```python
from build123d import *

# Parameters (mm, degrees)
F1_DEPTH = 6.858


with BuildPart() as f1:
    # F0 (on Front) → F1 (new body)
    with BuildSketch(Plane.XZ):
        with BuildLine():
            Line((28.575, 3.175), (0, 3.175))
            Line((0, 3.175), (-28.575, 3.175))
            ThreePointArc((-28.575, 3.175), (-48.6519, 5.867462), (-67.31, 13.754578))
            Line((-67.31, 13.754578), (-91.44, 13.754578))
            Line((-91.44, 13.754578), (-91.44, -13.754578))
            Line((-91.44, -13.754578), (-67.31, -13.754578))
            ThreePointArc((-67.31, -13.754578), (-48.6519, -5.867462), (-28.575, -3.175))
            Line((-28.575, -3.175), (0, -3.175))
            Line((0, -3.175), (28.575, -3.175))
            ThreePointArc((28.575, -3.175), (48.6519, -5.867462), (67.31, -13.754578))
            Line((67.31, -13.754578), (91.44, -13.754578))
            Line((91.44, -13.754578), (91.44, 13.754578))
            Line((91.44, 13.754578), (67.31, 13.754578))
            ThreePointArc((67.31, 13.754578), (48.6519, 5.867462), (28.575, 3.175))
        make_face()
    extrude(amount=F1_DEPTH)


solid = f1.part
```
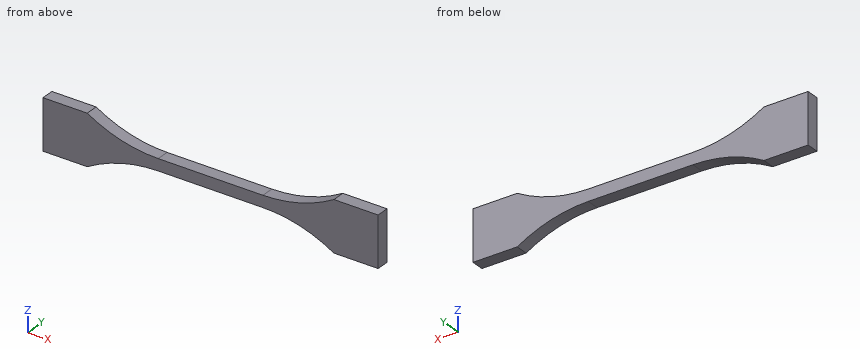
CAD build for the part. Positions are in the model's coordinates, mm. Round coordinates to 2 decimals unless told otherwise and drop trailing zeros. Loops run counter-clockwise (first coordinate to the right, second up) from the corner with the lowest first, then second, coordinate; pieces in that order, holes last. Notation, with made-up numbers: M 40,-32.5 L 88,-32.5 A23 ccw 88,-5.5 Z; hole C 10.25,-23 d8. An arc over 180 degrees is marked long. Return JSON: item names as keys, results as strings. Group by question number.
(1) Saw through at C-C, the plane x = -18. List the corners of the cut face in (y, z) (3 decimals).
(2) Drop flat-ended pins along their axis: P1, Ø1, axis at x = -2, z = 3.5, coming from the +Y side; P2, Ø10, axis at x = 37, z = -10, coming from the -Y side; P3, Ø4, axis at x = 11.5, y = -2.5, coming from the -Z side (3 decimals). Give the stop position or say it passes through.
(3) Saw through at D-D, the plane z = -10.5. List the corners of the cut face in (x, y), and give its area (3 significant figures).
(4) Saw through at A-A, the plane z = 8.5. List the corners of the cut face in (x, y), and give its area (3 significant figures).
(5) Wall check: probe 1 along X at (y, z) = (-1.5, -9.5); probe 2 along X at (y, z) = (-1.5, 10.75); probe 3 along Z at (x, y) = (15, -0.75) (3 decimals). Give the ranges that are in metal, low to high. Write a range as [from, to].
(6) Saw through at B-B, the plane y = -1.25. List the corners of the cut face in (x, z) (3 decimals), and give its area (3 significant figures).
Answer list:
{
 "1": {"outline": "M -6.858,-3.175 L 0,-3.175 L 0,3.175 L -6.858,3.175 Z"},
 "2": {"P1": "y = 0", "P2": "through", "P3": "z = -3.175"},
 "3": {"outline": "M -91.44,-6.86 L -61.17,-6.86 L -61.17,0 L -91.44,0 Z; M 61.17,-6.86 L 91.44,-6.86 L 91.44,0 L 61.17,0 Z", "area": "415 mm2"},
 "4": {"outline": "M -91.44,-6.86 L -56.56,-6.86 L -56.56,0 L -91.44,0 Z; M 56.56,-6.86 L 91.44,-6.86 L 91.44,0 L 56.56,0 Z", "area": "478 mm2"},
 "5": {"probe 1": "[-91.44, -58.97], [58.97, 91.44]", "probe 2": "[-91.44, -61.7], [61.7, 91.44]", "probe 3": "[-3.175, 3.175]"},
 "6": {"outline": "M -91.44,-13.755 L -67.31,-13.755 A76.2 cw -28.575,-3.175 L 28.575,-3.175 A76.2 cw 67.31,-13.755 L 91.44,-13.755 L 91.44,13.755 L 67.31,13.755 A76.2 cw 28.575,3.175 L -28.575,3.175 A76.2 cw -67.31,13.755 L -91.44,13.755 Z", "area": "2,710 mm2"}
}
